```python
from build123d import *

# Parameters (mm, degrees)
F0_W     = 76.094658
F0_H     = 76.094658
F1_DEPTH = 76.0984
F3_DEPTH = 76.0984
F4_R     = 23.46217
F5_DEPTH = 63.5


with BuildPart() as f1:
    # F0 (on Front) → F1 (new body)
    with BuildSketch(Plane.XZ):
        Rectangle(F0_W, F0_H)
    extrude(amount=F1_DEPTH)

    # F2 (on face) → F3 (cut)
    with BuildSketch(Plane(origin=(-38.047329, 0, 0), x_dir=(0, -1, 0), z_dir=(-1, 0, 0))):
        Polygon((76.0984, -38.047329), (0, 38.047329), (0, -38.047329), align=None)
    extrude(amount=-F3_DEPTH, mode=Mode.SUBTRACT)

    # F4 (on face) → F5 (cut)
    with BuildSketch(Plane.XZ.offset(76.0984)):
        Circle(F4_R)
    extrude(amount=-F5_DEPTH, mode=Mode.SUBTRACT)


solid = f1.part
```
Build history of the part. All positions in model axes, mm. Give positions to 0.01 mm unless a question says otherwise; leave off trailing zeros. Loops run counter-clockwise (first coordinate to the right, second up) from the corner with the lowest first, then second, coordinate; pieces in that order, holes last.
1) Drop flat-ended pins along their axis: P1, Ø1, axis at x = -25, y = -47.5, coming from the -Z side; P2, Ø8, axis at x = -22, z = 24.5, coming from the +Y side; P3, Ø2, axis at x = -26, z = 9.5, coming from the +Y side. Give the stop position or say it passes through.
Values follow:
P1: stops at z = -9.95
P2: stops at y = -9.55
P3: stops at y = -27.55
2) Band-saw the part on B-B on z = 12.5. List the corners of the cut face in (x, y).
Values follow:
outline: (-38.05, -76.1) - (-19.86, -76.1) - (-19.86, -25.55) - (-38.05, -25.55) - close; (19.86, -76.1) - (38.05, -76.1) - (38.05, -25.55) - (19.86, -25.55) - close
3) Probe line 1 along X through (y, z) = (-59.5, 0); line 2 along Z through (x, y) = (0, -47); line 3 along Z through (x, y) = (0, -62). List the from-to ranges inside material, lowest first.
Values follow:
line 1: x = -38.05 to -23.46, 23.46 to 38.05
line 2: z = 23.46 to 38.05
line 3: z = -23.95 to -23.46, 23.46 to 38.05
4) Band-saw the part on C-C on y = -66. List the corners of the cut face in (x, z).
Values follow:
outline: (-38.05, -27.95) - (38.05, -27.95) - (38.05, 38.05) - (-38.05, 38.05) - close; hole circle Ø46.92 at (0, 0)
5) Band-saw the part on D-D on x = 0. List the corners of the cut face in (y, z), then the cut area to 3 significant figures.
Values follow:
outline: (-76.1, -38.05) - (-61.51, -23.46) - (-76.1, -23.46) - close; (-76.1, 23.46) - (-14.59, 23.46) - (0, 38.05) - (-76.1, 38.05) - close
area: 1,110 mm2
6) Two-plate mould, pull along X, no slides. Class faces 1 (the face through (-1, -38, 38.047)), 2 (the face through (-38.047, -54, 16)), 3 (the face through (-3.054, -52.607, 23.263)), 4 (the face through (38.047, -54, 16)): released by +X, released by -X, zero draft, split by the parting line, or undercut.
Values follow:
face 1: zero draft
face 2: released by -X
face 3: undercut
face 4: released by +X
7) Band-saw the part on A-A on x = -14. List the corners of the cut face in (y, z), then the cut area to 3 significant figures.
Values follow:
outline: (-76.1, -38.05) - (-56.88, -18.83) - (-76.1, -18.83) - close; (-76.1, 18.83) - (-19.22, 18.83) - (0, 38.05) - (-76.1, 38.05) - close
area: 1,460 mm2
